```python
from build123d import *

# Parameters (mm, degrees)
SKETCH_R        = 5
SKETCH_R_2      = 3.2
PAD_DEPTH       = 15
SKETCH002_R     = 6.1
POCKET001_DEPTH = 4
SKETCH003_R     = 11.1
POCKET_DEPTH    = 7.4
FILLET_R        = 4
CHAMFER_SIZE    = 0.4
CHAMFER001_SIZE = 0.4


with BuildPart() as part:
    # Sketch → Pad (new body)
    with BuildSketch(Plane.XY):
        Polygon((20, 30), (20, 50.15), (62.3, 50.15), (62.3, 30), (82.3, 30), (82.3, 0), (0, 0), (0, 30), align=None)
        with Locations((41.15, 29)):
            Circle(SKETCH_R, mode=Mode.SUBTRACT)
        with Locations((11.15, 10)):
            Circle(SKETCH_R_2, mode=Mode.SUBTRACT)
        with Locations((31.15, 10)):
            Circle(SKETCH_R_2, mode=Mode.SUBTRACT)
        with Locations((51.15, 10)):
            Circle(SKETCH_R_2, mode=Mode.SUBTRACT)
        with Locations((71.15, 10)):
            Circle(SKETCH_R_2, mode=Mode.SUBTRACT)
    extrude(amount=PAD_DEPTH)

    # Sketch002 → Pocket001 (cut)
    with BuildSketch(Plane(origin=(0, 0, 0), x_dir=(1, 0, 0), z_dir=(0, 0, -1))):
        with Locations((11.15, -10)):
            Circle(SKETCH002_R)
        with Locations((31.15, -10)):
            Circle(SKETCH002_R)
        with Locations((51.15, -10)):
            Circle(SKETCH002_R)
        with Locations((71.15, -10)):
            Circle(SKETCH002_R)
    extrude(amount=-POCKET001_DEPTH, mode=Mode.SUBTRACT)

    # Sketch003 (on Face5 of Pocket001) → Pocket (cut)
    with BuildSketch(Plane.XY.offset(15)):
        with Locations((41.15, 29)):
            Circle(SKETCH003_R)
    extrude(amount=-POCKET_DEPTH, mode=Mode.SUBTRACT)

    # Fillet
    fillet_edges = [part.edges().sort_by_distance(p)[0] for p in [
        (82.3, 0, 7.5),
        (0, 0, 7.5),
        (0, 30, 7.5),
        (20, 30, 7.5),
        (20, 50.15, 7.5),
        (62.3, 50.15, 7.5),
        (62.3, 30, 7.5),
        (82.3, 30, 7.5),
    ]]
    fillet(fillet_edges, radius=FILLET_R)

    # Chamfer
    chamfer_edges = [part.edges().sort_by_distance(p)[0] for p in [
        (20, 40.075, 15),
        (18.828427, 31.171573, 15),
        (21.171573, 48.978427, 15),
        (10, 30, 15),
        (41.15, 50.15, 15),
        (1.171573, 28.828427, 15),
        (61.128427, 48.978427, 15),
        (0, 15, 15),
        (62.3, 40.075, 15),
        (1.171573, 1.171573, 15),
        (63.471573, 31.171573, 15),
        (41.15, 0, 15),
        (72.3, 30, 15),
        (81.128427, 1.171573, 15),
        (81.128427, 28.828427, 15),
        (82.3, 15, 15),
        (67.95, 10, 15),
        (47.95, 10, 15),
        (27.95, 10, 15),
        (7.95, 10, 15),
        (30.05, 29, 15),
    ]]
    chamfer(chamfer_edges, length=CHAMFER_SIZE)

    # Chamfer001
    chamfer001_edges = [part.edges().sort_by_distance(p)[0] for p in [
        (20, 40.075, 0),
        (18.828427, 31.171573, 0),
        (21.171573, 48.978427, 0),
        (10, 30, 0),
        (41.15, 50.15, 0),
        (1.171573, 28.828427, 0),
        (61.128427, 48.978427, 0),
        (0, 15, 0),
        (62.3, 40.075, 0),
        (1.171573, 1.171573, 0),
        (63.471573, 31.171573, 0),
        (41.15, 0, 0),
        (72.3, 30, 0),
        (81.128427, 1.171573, 0),
        (81.128427, 28.828427, 0),
        (82.3, 15, 0),
        (65.05, 10, 0),
        (45.05, 10, 0),
        (25.05, 10, 0),
        (5.05, 10, 0),
        (36.15, 29, 0),
    ]]
    chamfer(chamfer001_edges, length=CHAMFER001_SIZE)


solid = part.part
```
Input: part model. Units: mm. Frame: model coordinates. A direction names the side the tool comes from. Give positions to 0.01 mm unless a question says otherwise; leave off trailing zeros. Write each loop counter-clockwise with the first axis right and the second up, starting at its lowest first coordinate (ties: lowest second). Pieces come first, ordered by that corner, then holes. Notation, with made-up numbers: (-26, 75) - (3, 75) arc R15 ccw to (3, 89) - close; hole circle Ø1 at (-21.5, 53.5). An arc over 180 degrees is marked (long way). Write item = value, one per line. Start each with the question number.
1. Section query D-D, the plane x = 71.15. Output: boundary loops of the cut face in (y, z).
2. Ray query, L1, parallel to X at y = 10, z = 12.75; L2, parallel to X at y = 10, z = 1.35; L3, parallel to Y at x = 71.15, z = 2.3. Return the intervals inside material, ascending.
3. Section query C-C, the plane y = 10. Count the separate pieces of the cut face and the enclosed holes in it, then the cut area to 3 significant figures.
4. Access query for faces 1 (the conical face through (80.893, 28.651, 0.108)), 2 (the flat face through (62.3, 40, 7)), 3 (the cylindrical face through (9.828, 15.955, 2.175)). Directions: +Z, -Z, +X, -X, +Y, -Y. A direction counts if a zero-diameter tool reaches every point of the face in a straight line with its end or side. Return the directions, or none.
5. Section query A-A, the plane z = 9.5. Output: boundary loops of the cut face in (x, y), then the cut area to 3 significant figures.
6. Mould query, pull axis X, two halves, no side actions, for faces 4 (the cylindrical face through (63.441, 31.203, 7.599)), 5 (the flat face through (54, 13, 4)), 6 (the cylindrical face through (21.141, 48.947, 7.599)). Classes: released by +X, released by -X, zero draft, split by the parting line, or undercut.
7. First-contact query: pin 1 Ø6 at (y, z) = (40.5, 6) entering from -X; pin 2 Ø18 at (x, y) = (40, 29.5) entering from +Z; pin 3 Ø6 at (x, z) = (7, 8.5) entering from +Y; pin 4 Ø6 at (x, y) = (31.15, 10) entering from -Z. Flat tips, straight axial feed; report the tip coordinate or a pass-through.
8. Section query B-B, the plane x = 41.15. Output: boundary loops of the cut face in (y, z).
Check sheet entries:
q1.outline = (0, 0.4) - (0.4, 0) - (3.5, 0) - (3.9, 0.4) - (3.9, 4) - (6.8, 4) - (6.8, 14.6) - (6.4, 15) - (0.4, 15) - (0, 14.6) - close; (13.2, 4) - (16.1, 4) - (16.1, 0.4) - (16.5, 0) - (29.6, 0) - (30, 0.4) - (30, 14.6) - (29.6, 15) - (13.6, 15) - (13.2, 14.6) - close
q2.L1 = 0 to 7.95, 14.35 to 27.95, 34.35 to 47.95, 54.35 to 67.95, 74.35 to 82.3
q2.L2 = 0 to 5.05, 17.25 to 25.05, 37.25 to 45.05, 57.25 to 65.05, 77.25 to 82.3
q2.L3 = 0 to 3.9, 16.1 to 30
q3.separate_pieces = 5
q3.enclosed_holes = 0
q3.area = 756 mm2
q4.face_1 = -Z, +X, +Y
q4.face_2 = +Z, -Z, +X, +Y
q4.face_3 = -Z
q5.outline = (0, 4) arc R4 ccw to (4, 0) - (78.3, 0) arc R4 ccw to (82.3, 4) - (82.3, 26) arc R4 ccw to (78.3, 30) - (66.3, 30) arc R4 cw to (62.3, 34) - (62.3, 46.15) arc R4 ccw to (58.3, 50.15) - (24, 50.15) arc R4 ccw to (20, 46.15) - (20, 34) arc R4 cw to (16, 30) - (4, 30) arc R4 ccw to (0, 26) - close; hole circle Ø6.4 at (11.15, 10); hole circle Ø6.4 at (31.15, 10); hole circle Ø22.2 at (41.15, 29); hole circle Ø6.4 at (51.15, 10); hole circle Ø6.4 at (71.15, 10)
q5.area = 2,790 mm2
q6.face_4 = released by +X
q6.face_5 = undercut
q6.face_6 = released by -X
q7.pin_1 = 20
q7.pin_2 = 7.6
q7.pin_3 = 30
q7.pin_4 = through
q8.outline = (0, 0.4) - (0.4, 0) - (23.6, 0) - (24, 0.4) - (24, 7.6) - (17.9, 7.6) - (17.9, 14.6) - (17.5, 15) - (0.4, 15) - (0, 14.6) - close; (34, 0.4) - (34.4, 0) - (49.75, 0) - (50.15, 0.4) - (50.15, 14.6) - (49.75, 15) - (40.5, 15) - (40.1, 14.6) - (40.1, 7.6) - (34, 7.6) - close
